Input: part model. Units: mm. Frame: model coordinates. Face numbers are marked on the shaded views. A direction names the side the tool comes from. Give positions to 0.01 mm unless a question says otherwise; leave off trailing zeros. Loops run counter-clockwise (first coordinate to the right, second up) from the corner with the lowest first, then second, coordinate; pieces in that order, holes last. Notation, with made-up numbers: M 5.5,51.25 L 36.5,51.25 A16 cw 36.5,60.25 Z; hole C -23,84.5 d9. An arc over 180 degrees is marked long. Use CSV: the item, a comma, the result in double quotes. Start each with the question number.
Q1. Material intervals for line 1 along Y through (x, z) = (50.5, 15.5); line 2 along X through (y, z) = (51, 11.5); line 3 along X through (y, z) = (17.5, 5.75), sorted ascending.
Q2. Reachability of the marked faces 1, 2, 3 and 4 from +Z, -Z, +X, -X, +Y, -Y: full face, straight path, thin tool, end or side. Return the list, or none.
Q3. Pin query (flat end, axial travel): pin 1 (12 mm diameter, centred on y = 20, z = 15.5, fed in from +X); pin 2 (4 mm diameter, centred on y = 33.5, z = 13, fed in from +X); pin 3 (1.5 mm diameter, centred on y = -2, z = 14, fed in from +X). Return the tip coordinate at first contact, or that it passes through.
Q4. Section A-A, the plane y = 0. Output: boundary loops of the cut face in (x, z), plus the area to 3 significant figures.
Q5. Section B-B, the plane x = -12. Output: boundary loops of the cut face in (y, z), plus the area to 3 significant figures.
Q6. Pull-direction query (Y, two-part tool) for the marked faces 5, 6, 7 and 8; classes: released by +Y, released by -Y, zero draft, split by the parting line, or undercut.
from build123d import *

# Parameters (mm, degrees)
SKETCH1_R           = 30
BOSS_EXTRUDE1_DEPTH = 20
FILLET1_R           = 3


with BuildPart() as part:
    # Sketch1 → Boss-Extrude1 (new body)
    with BuildSketch(Plane.XY):
        with BuildLine():
            ThreePointArc((0, 60), (-2.617163242, 59.942893295), (-5.229344565, 59.771681886))
            Line((-5.229344565, 59.771681886), (-8.682408883, 49.240387651))
            ThreePointArc((-8.682408883, 49.240387651), (-12.940952255, 48.296291314), (-17.101007166, 46.984631039))
            Line((-17.101007166, 46.984631039), (-25.357095704, 54.378467222))
            ThreePointArc((-25.357095704, 54.378467222), (-30, 51.961524227), (-34.414586181, 49.149122657))
            Line((-34.414586181, 49.149122657), (-32.139380484, 38.302222156))
            ThreePointArc((-32.139380484, 38.302222156), (-35.355339059, 35.355339059), (-38.302222156, 32.139380484))
            Line((-38.302222156, 32.139380484), (-49.149122657, 34.414586181))
            ThreePointArc((-49.149122657, 34.414586181), (-51.961524227, 30), (-54.378467222, 25.357095704))
            Line((-54.378467222, 25.357095704), (-46.984631039, 17.101007166))
            ThreePointArc((-46.984631039, 17.101007166), (-48.296291314, 12.940952255), (-49.240387651, 8.682408883))
            Line((-49.240387651, 8.682408883), (-59.771681886, 5.229344565))
            ThreePointArc((-59.771681886, 5.229344565), (-60, 0), (-59.771681886, -5.229344565))
            Line((-59.771681886, -5.229344565), (-49.240387651, -8.682408883))
            ThreePointArc((-49.240387651, -8.682408883), (-48.296291314, -12.940952255), (-46.984631039, -17.101007166))
            Line((-46.984631039, -17.101007166), (-54.378467222, -25.357095704))
            ThreePointArc((-54.378467222, -25.357095704), (-51.961524227, -30), (-49.149122657, -34.414586181))
            Line((-49.149122657, -34.414586181), (-38.302222156, -32.139380484))
            ThreePointArc((-38.302222156, -32.139380484), (-35.355339059, -35.355339059), (-32.139380484, -38.302222156))
            Line((-32.139380484, -38.302222156), (-34.414586181, -49.149122657))
            ThreePointArc((-34.414586181, -49.149122657), (-30, -51.961524227), (-25.357095704, -54.378467222))
            Line((-25.357095704, -54.378467222), (-17.101007166, -46.984631039))
            ThreePointArc((-17.101007166, -46.984631039), (-12.940952255, -48.296291314), (-8.682408883, -49.240387651))
            Line((-8.682408883, -49.240387651), (-5.229344565, -59.771681886))
            ThreePointArc((-5.229344565, -59.771681886), (0, -60), (5.229344565, -59.771681886))
            Line((5.229344565, -59.771681886), (8.682408883, -49.240387651))
            ThreePointArc((8.682408883, -49.240387651), (12.940952255, -48.296291314), (17.101007166, -46.984631039))
            Line((17.101007166, -46.984631039), (25.357095704, -54.378467222))
            ThreePointArc((25.357095704, -54.378467222), (30, -51.961524227), (34.414586181, -49.149122657))
            Line((34.414586181, -49.149122657), (32.139380484, -38.302222156))
            ThreePointArc((32.139380484, -38.302222156), (35.355339059, -35.355339059), (38.302222156, -32.139380484))
            Line((38.302222156, -32.139380484), (49.149122657, -34.414586181))
            ThreePointArc((49.149122657, -34.414586181), (51.961524227, -30), (54.378467222, -25.357095704))
            Line((54.378467222, -25.357095704), (46.984631039, -17.101007166))
            ThreePointArc((46.984631039, -17.101007166), (48.296291314, -12.940952255), (49.240387651, -8.682408883))
            Line((49.240387651, -8.682408883), (59.771681886, -5.229344565))
            ThreePointArc((59.771681886, -5.229344565), (60, 0), (59.771681886, 5.229344565))
            Line((59.771681886, 5.229344565), (49.240387651, 8.682408883))
            ThreePointArc((49.240387651, 8.682408883), (48.296291314, 12.940952255), (46.984631039, 17.101007166))
            Line((46.984631039, 17.101007166), (54.378467222, 25.357095704))
            ThreePointArc((54.378467222, 25.357095704), (51.961524227, 30), (49.149122657, 34.414586181))
            Line((49.149122657, 34.414586181), (38.302222156, 32.139380484))
            ThreePointArc((38.302222156, 32.139380484), (35.355339059, 35.355339059), (32.139380484, 38.302222156))
            Line((32.139380484, 38.302222156), (34.414586181, 49.149122657))
            ThreePointArc((34.414586181, 49.149122657), (30, 51.961524227), (25.357095704, 54.378467222))
            Line((25.357095704, 54.378467222), (17.101007166, 46.984631039))
            ThreePointArc((17.101007166, 46.984631039), (12.940952255, 48.296291314), (8.682408883, 49.240387651))
            Line((8.682408883, 49.240387651), (5.229344565, 59.771681886))
            ThreePointArc((5.229344565, 59.771681886), (2.617163242, 59.942893295), (0, 60))
        make_face()
        Circle(SKETCH1_R, mode=Mode.SUBTRACT)
    extrude(amount=BOSS_EXTRUDE1_DEPTH)

    # Fillet1
    fillet1_edges = [part.edges().sort_by_distance(p)[0] for p in [
        (-34.414586181, 49.149122657, 10),
        (-25.357095704, 54.378467222, 10),
        (-17.101007166, 46.984631039, 10),
        (-8.682408883, 49.240387651, 10),
        (-5.229344565, 59.771681886, 10),
        (5.229344565, 59.771681886, 10),
        (8.682408883, 49.240387651, 10),
        (17.101007166, 46.984631039, 10),
        (25.357095704, 54.378467222, 10),
        (34.414586181, 49.149122657, 10),
        (32.139380484, 38.302222156, 10),
        (38.302222156, 32.139380484, 10),
        (49.149122657, 34.414586181, 10),
        (54.378467222, 25.357095704, 10),
        (46.984631039, 17.101007166, 10),
        (49.240387651, 8.682408883, 10),
        (59.771681886, 5.229344565, 10),
        (59.771681886, -5.229344565, 10),
        (49.240387651, -8.682408883, 10),
        (46.984631039, -17.101007166, 10),
        (54.378467222, -25.357095704, 10),
        (49.149122657, -34.414586181, 10),
        (38.302222156, -32.139380484, 10),
        (32.139380484, -38.302222156, 10),
        (34.414586181, -49.149122657, 10),
        (25.357095704, -54.378467222, 10),
        (17.101007166, -46.984631039, 10),
        (8.682408883, -49.240387651, 10),
        (5.229344565, -59.771681886, 10),
        (-5.229344565, -59.771681886, 10),
        (-8.682408883, -49.240387651, 10),
        (-17.101007166, -46.984631039, 10),
        (-25.357095704, -54.378467222, 10),
        (-34.414586181, -49.149122657, 10),
        (-32.139380484, -38.302222156, 10),
        (-38.302222156, -32.139380484, 10),
        (-49.149122657, -34.414586181, 10),
        (-54.378467222, -25.357095704, 10),
        (-46.984631039, -17.101007166, 10),
        (-49.240387651, -8.682408883, 10),
        (-59.771681886, -5.229344565, 10),
        (-59.771681886, 5.229344565, 10),
        (-49.240387651, 8.682408883, 10),
        (-46.984631039, 17.101007166, 10),
        (-54.378467222, 25.357095704, 10),
        (-49.149122657, 34.414586181, 10),
        (-38.302222156, 32.139380484, 10),
        (-32.139380484, 38.302222156, 10),
    ]]
    fillet(fillet1_edges, radius=FILLET1_R)


solid = part.part
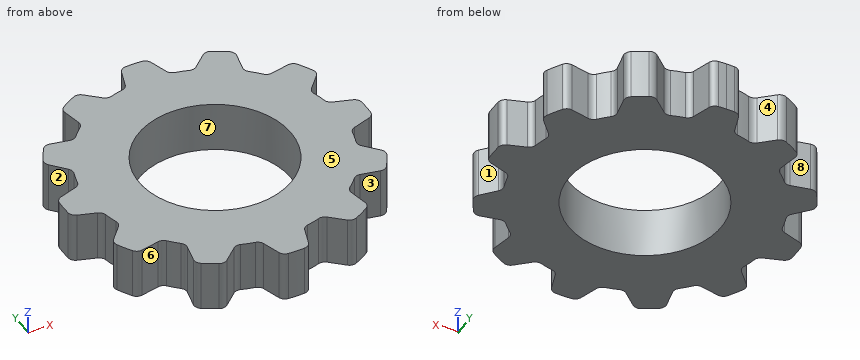
A:
1,line 1,"-32.4 to -21.03, -8.3 to 8.3, 21.03 to 32.4"
1,line 2,"-31.61 to -21.58, -8.11 to 8.11, 21.58 to 31.61"
1,line 3,"-47.6 to -24.37, 24.37 to 47.6"
2,face 1,"+Z, -Z, +X"
2,face 2,"+Z, -Z, -X"
2,face 3,"+Z, -Z, -Y"
2,face 4,"+Z, -Z, +Y"
3,pin 1,"x = 53.8"
3,pin 2,"x = 51.07"
3,pin 3,"x = 59.99"
4,outline,"M -60,0 L -30,0 L -30,20 L -60,20 Z; M 30,0 L 60,0 L 60,20 L 30,20 Z"
4,area,"1,200 mm^2"
5,outline,"M -48.54,0 L -27.5,0 L -27.5,20 L -48.54,20 Z; M 27.5,0 L 48.54,0 L 48.54,20 L 27.5,20 Z"
5,area,"842 mm^2"
6,face 5,"zero draft"
6,face 6,"released by -Y"
6,face 7,"undercut"
6,face 8,"released by +Y"
